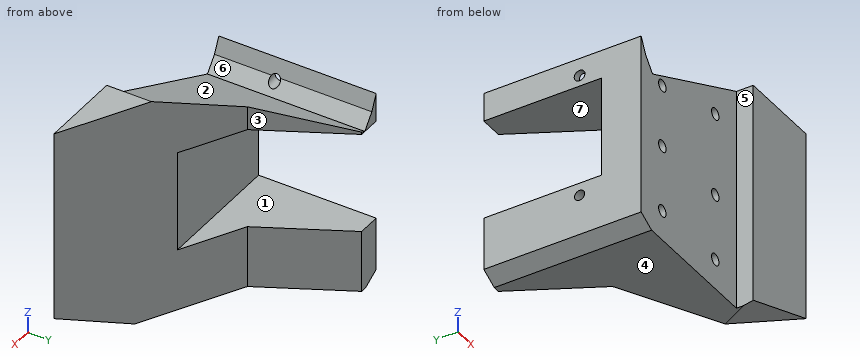
```python
from build123d import *

# Parameters (mm, degrees)
CROQUIS1_W              = 67
CROQUIS1_H              = 51.82
SALIENTE_EXTRUIR1_DEPTH = 70
CORTAR_EXTRUIR1_REACH   = 69
CROQUIS4_W              = 60
CROQUIS4_H              = 30
CORTAR_EXTRUIR2_DEPTH   = 35
CORTAR_EXTRUIR3_REACH   = 69
CROQUIS5_W              = 45
CROQUIS5_H              = 5
CORTAR_EXTRUIR4_REACH   = 53.82
CORTAR_EXTRUIR5_REACH   = 53.82
CROQUIS9_R              = 1.6
CROQUIS9_R_2            = 1.522094027
CORTAR_EXTRUIR6_DEPTH   = 6
CROQUIS11_R             = 1.75
CORTAR_EXTRUIR7_DEPTH   = 6
CORTAR_EXTRUIR8_REACH   = 34.863


with BuildPart() as part:
    # Croquis1 → Saliente-Extruir1 (new body)
    with BuildSketch(Plane(origin=(0, 0, 0), x_dir=(0, 0, -1), z_dir=(1, 0, 0))):
        with Locations((33.5, 25.91)):
            Rectangle(CROQUIS1_W, CROQUIS1_H)
    extrude(amount=SALIENTE_EXTRUIR1_DEPTH)

    # Croquis3 → Cortar-Extruir1 (cut, up to next)
    with BuildSketch(Plane.XY, mode=Mode.PRIVATE) as cortar_extruir1_sk1:
        Polygon((70, 0), (20.404370982, 26.370463718), (6.872612509, 51.82), (70, 51.82), align=None)
    cortar_extruir1_tool1 = extrude(cortar_extruir1_sk1.sketch, amount=-CORTAR_EXTRUIR1_REACH, mode=Mode.PRIVATE) & part.part
    add(cortar_extruir1_tool1.solids().sort_by_distance((45.373987, 32.707801, 0))[0], mode=Mode.SUBTRACT)

    # Croquis4 → Cortar-Extruir2 (cut)
    with BuildSketch(Plane(origin=(0, 51.82, 0), x_dir=(1, 0, 0), z_dir=(0, 1, 0))):
        with Locations((30, 33.5)):
            Rectangle(CROQUIS4_W, CROQUIS4_H)
    extrude(amount=-CORTAR_EXTRUIR2_DEPTH, mode=Mode.SUBTRACT)

    # Croquis5 → Cortar-Extruir3 (cut, up to next)
    with BuildSketch(Plane.XY, mode=Mode.PRIVATE) as cortar_extruir3_sk1:
        with Locations((22.5, 2.5)):
            Rectangle(CROQUIS5_W, CROQUIS5_H)
    cortar_extruir3_tool1 = extrude(cortar_extruir3_sk1.sketch, amount=-CORTAR_EXTRUIR3_REACH, mode=Mode.PRIVATE) & part.part
    add(cortar_extruir3_tool1.solids().sort_by_distance((22.5, 2.5, 0))[0], mode=Mode.SUBTRACT)

    # Croquis6 → Cortar-Extruir4 (cut, up to next)
    with BuildSketch(Plane(origin=(0, 51.82, 0), x_dir=(1, 0, 0), z_dir=(0, 1, 0)), mode=Mode.PRIVATE) as cortar_extruir4_sk1:
        Polygon((4.922856145, 67), (0, 64.334655313), (0, 67), align=None)
    cortar_extruir4_tool1 = extrude(cortar_extruir4_sk1.sketch, amount=-CORTAR_EXTRUIR4_REACH, mode=Mode.PRIVATE) & part.part
    add(cortar_extruir4_tool1.solids().sort_by_distance((1.640952, 51.82, -66.111552))[0], mode=Mode.SUBTRACT)

    # Croquis8 → Cortar-Extruir5 (cut, up to next)
    with BuildSketch(Plane(origin=(0, 51.82, 0), x_dir=(1, 0, 0), z_dir=(0, 1, 0)), mode=Mode.PRIVATE) as cortar_extruir5_sk1:
        Polygon((45, 0), (5.376842989, 18.476581555), (2.059345913, 14.392541381), (0, 9.976259819), (0, -0.062203445), (6.872612509, 0), (20.404370982, 0), align=None)
    cortar_extruir5_tool1 = extrude(cortar_extruir5_sk1.sketch, amount=-CORTAR_EXTRUIR5_REACH, mode=Mode.PRIVATE) & part.part
    add(cortar_extruir5_tool1.solids().sort_by_distance((15.782883, 51.82, -6.412773))[0], mode=Mode.SUBTRACT)

    # Croquis9 → Cortar-Extruir6 (cut)
    with BuildSketch(Plane.ZY):
        with Locations((-15.25, 23.32)):
            Circle(CROQUIS9_R)
        with Locations((-52.25, 23.32)):
            Circle(CROQUIS9_R_2)
    extrude(amount=-CORTAR_EXTRUIR6_DEPTH, mode=Mode.SUBTRACT)

    # Croquis11 → Cortar-Extruir7 (cut)
    with BuildSketch(Plane.XZ.offset(-5)):
        with Locations((35, -58)):
            Circle(CROQUIS11_R)
        with Locations((10, -58)):
            Circle(CROQUIS11_R)
        with Locations((10, -38)):
            Circle(CROQUIS11_R)
        with Locations((35, -38)):
            Circle(CROQUIS11_R)
        with Locations((10, -19.30137405)):
            Circle(CROQUIS11_R)
        with Locations((35, -13)):
            Circle(CROQUIS11_R)
    extrude(amount=-CORTAR_EXTRUIR7_DEPTH, mode=Mode.SUBTRACT)

    # Croquis13 → Cortar-Extruir8 (cut, up to next)
    with BuildSketch(Plane(origin=(15.428248379, 29.016315039, 0), x_dir=(0.882947593, -0.469471563, 0), z_dir=(0.469471563, 0.882947593, 0)), mode=Mode.PRIVATE) as cortar_extruir8_sk1:
        Polygon((34.467850213, 68.66403013), (75.183132097, 51.381418335), (75.183132097, 68.66403013), align=None)
    cortar_extruir8_tool1 = extrude(cortar_extruir8_sk1.sketch, amount=-CORTAR_EXTRUIR8_REACH, mode=Mode.PRIVATE) & part.part
    add(cortar_extruir8_tool1.solids().sort_by_distance((69.827861, 0.091528, -62.90316))[0], mode=Mode.SUBTRACT)


solid = part.part
```
CAD build for the part. Positions are in the model's coordinates, mm. Face numbers are marked on the shaded views. A direction names the side the tool comes from. Round coordinates to 2 decimals unless told otherwise and drop trailing zeros. Loops run counter-clockwise (first coordinate to the right, second up) from the corner with the lowest first, then second, coordinate; pieces in that order, holes last. Notation, with made-up numbers: M 33,-35.5 L 91,-35.5 A33 cw 91,-1.5 Z; hole C -18,59 d3. An arc over 180 degrees is marked long. Return JSON: item names as keys, results as strings. Group by question number.
(1) Drop flat-ended pins along their axis: P1, Ø3, axis at y = 33.5, z = -12.5, coming from the +X side; P2, Ø10, axis at x = 61, y = 6, coming from the -Z side; P3, Ø3, axis at x = 61, z = -16, coming from the +Y side. Give the stop position or say it passes through.
(2) Wall check: probe 1 along Z at (x, y) = (10, 7); probe 2 along Y at (x, z) = (4.25, -52.25); probe 3 along Y at (x, z) = (13, -31). Give the ranges that are in metal, low to high. Write a range as [from, to].
(3) Saw through at D-D, the plane y = 33. List the corners of the cut face in (x, z).
(4) Mould opens along X. For the marked faces 1, 2 and 3 say: +X half, -X half, draft (parallel to the pull), parting line (faces both ways), or undercut.
(5) Saw through at C-C, the plane x = 10. List the corners of the cut face in (y, z).
(6) Saw through at A-A, the plane y = 44. List the corners of the cut face in (x, z).
(7) Saw through at B-B, the plane z = -38. List the corners of the cut face in (x, y), and give its area (3 significant figures).
(8) Tool access for the marked faces 4, 5, 6 and 7: list every direction of +Z, -Z, +X, -X, +Y, -Y with a clear straight run to the whole face (end or side of a thin tool).
Answer list:
{
 "1": {"P1": "x = 17.39", "P2": "z = -63.7", "P3": "y = 5.58"},
 "2": {"probe 1": "[-67, -59.75], [-56.25, -39.75], [-36.25, -21.05], [-17.55, -16.32]", "probe 2": "[5, 21.8], [24.84, 51.82]", "probe 3": "[5, 16.82]"},
 "3": {"outline": "M 0,-64.33 L 4.92,-67 L 16.88,-67 L 16.88,-48.5 L 0,-48.5 Z; M 0,-18.5 L 16.88,-18.5 L 16.88,-13.11 L 5.38,-18.48 L 2.06,-14.39 L 0,-9.98 Z"},
 "4": {"face 1": "draft", "face 2": "undercut", "face 3": "+X half"},
 "5": {"outline": "M 5,-67 L 45.94,-67 L 45.94,-48.5 L 16.82,-48.5 L 16.82,-18.5 L 45.94,-18.5 L 45.94,-16.32 L 5,-16.32 L 5,-17.55 L 11,-17.55 L 11,-21.05 L 5,-21.05 L 5,-36.25 L 11,-36.25 L 11,-39.75 L 5,-39.75 L 5,-56.25 L 11,-56.25 L 11,-59.75 L 5,-59.75 Z"},
 "6": {"outline": "M 0,-64.33 L 4.92,-67 L 11.03,-67 L 11.03,-48.5 L 0,-48.5 Z; M 0,-18.5 L 11.03,-18.5 L 11.03,-15.84 L 5.38,-18.48 L 2.06,-14.39 L 0,-9.98 Z"},
 "7": {"outline": "M 0,5 L 8.25,5 L 8.25,11 L 11.75,11 L 11.75,5 L 33.25,5 L 33.25,11 L 36.75,11 L 36.75,5 L 45,5 L 45,0 L 70,0 L 38.37,16.82 L 0,16.82 Z", "area": "644 mm2"},
 "8": {"face 4": "-Z, +X, -X, +Y, -Y", "face 5": "+Z, -Z, -X, -Y", "face 6": "+Z, +Y, -Y", "face 7": "+X, -X, +Y"}
}
